Work out the finished part from the listing and answer in its coordinate system (mm). Face numbers are marked on the shaded views. A direction names the side the tool comes from. Give positions to 0.01 mm unless a question says otherwise; leave off trailing zeros. Write each loop counter-clockwise with the first axis right and the second up, starting at its lowest first coordinate (ties: lowest second). Pieces come first, ordered by that corner, then holes. Notation, with made-up numbers: (85.25, 66) -> (137.25, 66) arc R11 ccw to (137.25, 78) -> close; hole circle Ø5 at (-27.75, -19). An arc over 180 degrees is marked (long way). Use a Markdown table: item, result. Add a question column.
Q1. Section B-B, the plane y = -73.5 is taken. Give the vertices of the cut face in (x, z).
Q2. Section C-C, the plane z = 18.5 is taken. Give the vertices of the cut face in (x, y).
Q3. Section A-A, the plane z = 15.75 is taken. Give the vertices of the cut face in (x, y).
Q4. Each of these flat-tipped pins is pushed along its axis until it touches: pin 1 Ø6 at (x, z) = (6.5, 15) entering from -Y; pin 2 Ø3.5 at (x, z) = (-8, 13.5) entering from -Y. Where does it stop, or does it pass through?
Q5. For a pull along Z with two mould halves and no side action, classify the marked faces 3, 4 and 5 as pulls with the +Z half, pulls with the -Z half, needs draft (parallel to the pull), parting line crosses it, or undercut.
Q6. For the marked faces 1 and 2, determine the directions among +Z, -Z, +X, -X, +Y, -Y from which every point of the face is accessible in a straight line to the end or side of a thin tool.
Q7. Consider line 1 (Z direction, x = 2.5, y = -75.25); line 2 (X direction, y = -75, z = 17.5); line 3 (Z direction, x = 12.5, y = -77.75). Determine where each line is inside the solid, lowest interval first.
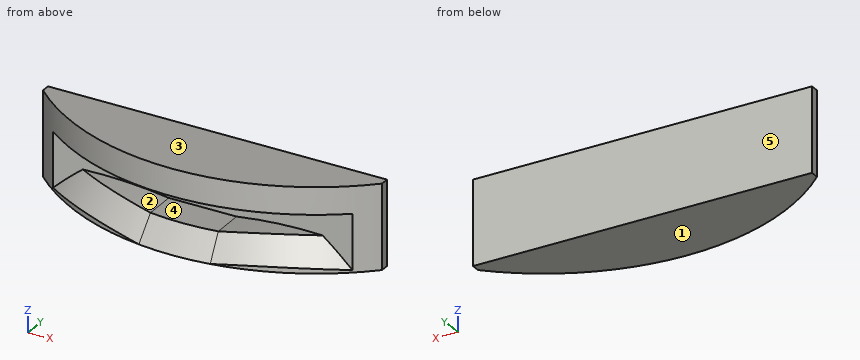
from build123d import *

# Parameters (mm, degrees)
PAD003_DEPTH    = 10
POCKET009_DEPTH = 6.001
CHAMFER_SIZE2   = 2
CHAMFER_SIZE    = 2.79


with BuildPart() as part:
    # Sketch036 → Pad003 (new body)
    with BuildSketch(Plane.XY):
        with BuildLine():
            ThreePointArc((-20, -1), (0, -9), (20, -1))
            Line((20, 0), (20, -1))
            Line((-20, 0), (20, 0))
            Line((-20, -1), (-20, 0))
        make_face()
    extrude(amount=PAD003_DEPTH)

    # Sketch037 (on DatumPlane) → Pocket009 (cut, through all)
    with BuildSketch(Plane.XZ.offset(3)):
        with BuildLine():
            Line((-20, 6.8), (20, 6.8))
            Line((20, 6.8), (20, 2.8))
            ThreePointArc((20, 2.8), (12, 3.4), (4, 2.8))
            Line((-4, 2.8), (4, 2.8))
            ThreePointArc((-4, 2.8), (-12, 3.4), (-20, 2.8))
            Line((-20, 2.8), (-20, 6.8))
        make_face()
    extrude(amount=POCKET009_DEPTH, mode=Mode.SUBTRACT)

    # Chamfer
    chamfer_edges = [part.edges().sort_by_distance(p)[0] for p in [
        (11.193894, -6.752509, 3.393942),
        (0, -9, 2.8),
        (-11.193894, -6.752509, 3.393942),
    ]]
    chamfer_side = part.faces().sort_by_distance((0, -9, 0.42))[0]
    chamfer(chamfer_edges, length=CHAMFER_SIZE, length2=CHAMFER_SIZE2, reference=chamfer_side)


with BuildPart() as part_1:
    # Body003 placement: moved
    add(part.part.moved(Location((0, -72, 10.5))))


solid = part_1.part
Result set:
| question | item | result |
|---|---|---|
| 1 | outline | (-19.46, 10.5) -> (19.46, 10.5) -> (19.46, 20.5) -> (-19.46, 20.5) -> close |
| 2 | outline | (-20, -73) arc R29 ccw to (20, -73) -> (20, -72) -> (-20, -72) -> close |
| 3 | outline | (-20, -73) arc R29 ccw to (-17.66, -75) -> (17.66, -75) arc R29 ccw to (20, -73) -> (20, -72) -> (-20, -72) -> close |
| 4 | pin 1 | stops at y = -80.64 |
| 4 | pin 2 | stops at y = -79.34 |
| 5 | face 3 | pulls with the +Z half |
| 5 | face 4 | undercut |
| 5 | face 5 | needs draft |
| 6 | face 1 | -Z, +X, -X, +Y, -Y |
| 6 | face 2 | -Y |
| 7 | line 1 | z = 10.5 to 13.3, 17.3 to 20.5 |
| 7 | line 2 | x = -17.66 to 17.66 |
| 7 | line 3 | z = 10.5 to 11.63, 17.3 to 20.5 |
